Can you work these out from the drawing? Everything is in mm from the part's minimum corner. Coordinates: 2 decimals unless noted, no trailing zeros. Loops run counter-clockwise (first coordinate to the right, second up) from the corner with the lowest first, then second, coordinate; pieces in that order, holes last.
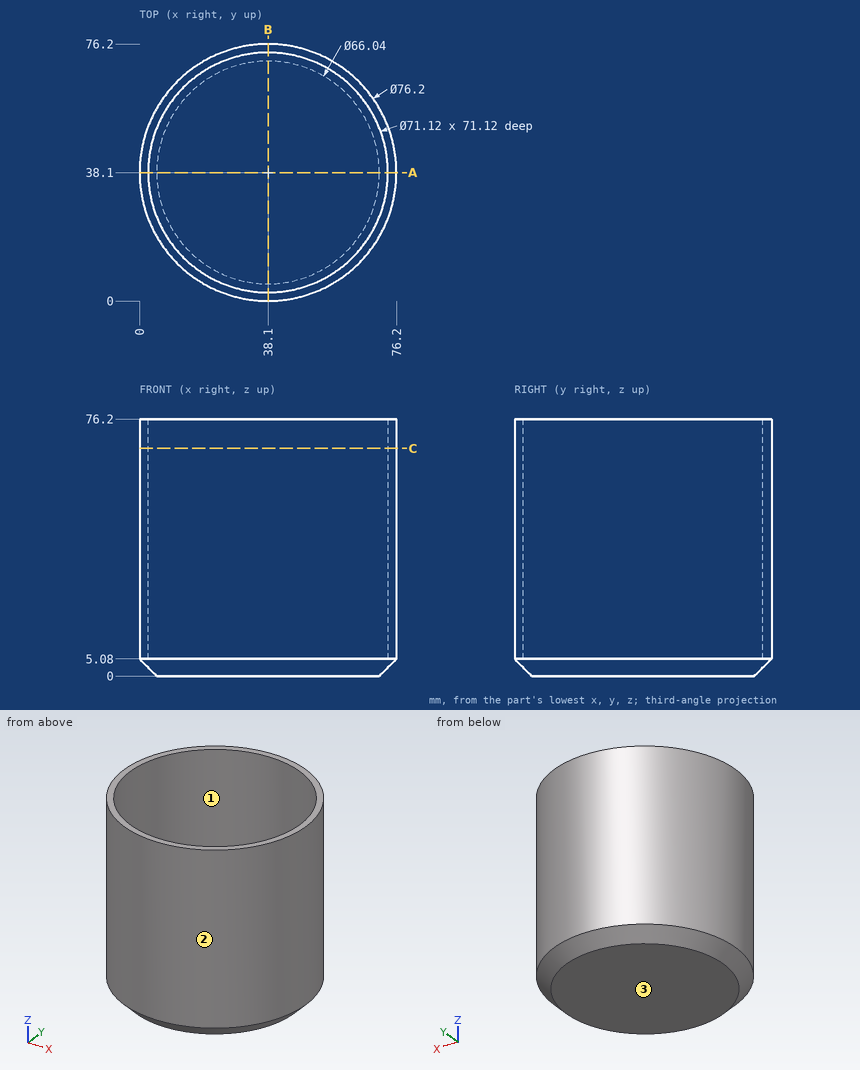
Item 1: Suppose I cut it at C-C, the plane z = 67.5. Please give me the cut outline in (x, y).
Results are:
outline: circle Ø76.2 at (38.1, 38.1); hole circle Ø71.12 at (38.1, 38.1)
Item 2: Suppose I cut it at A-A, the plane y = 38.1. Please give me the cut outline in (x, z).
Results are:
outline: (0, 5.08) - (5.08, 0) - (71.12, 0) - (76.2, 5.08) - (76.2, 76.2) - (73.66, 76.2) - (73.66, 5.08) - (2.54, 5.08) - (2.54, 76.2) - (0, 76.2) - close
Item 3: I'm going to push flat-ended pins straight in: P1, Ø4, axis at y = 56, z = 50, coming from the +X side; P2, Ø1.5, axis at x = 56.5, z = 12, coming from the -Y side; P3, Ø2, axis at x = 13, y = 11, coming from the -Z side. Where does each tip first touch, or does it pass through?
Results are:
P1: stops at x = 72.72
P2: stops at y = 4.33
P3: stops at z = 2.92
Item 4: We'd pull the mould along X, two halves only. Please class the marked faces 1, 2 and 3: +X half, -X half, draft (parallel to the pull), parting line (faces both ways), or undercut.
Results are:
face 1: undercut
face 2: parting line
face 3: draft
Item 5: I need wall thicknesses on line 1 along Y through (x, z) = (38, 58); line 2 along Z through (x, y) = (60.5, 43); line 3 along Y through (x, z) = (61.5, 49). Which ranges of each line are inside material? Lowest first, please.
Results are:
line 1: y = 0 to 2.54, 73.66 to 76.2
line 2: z = 0 to 5.08
line 3: y = 8.03 to 11.32, 64.88 to 68.17
